The drawing under review shows one solid part. Ordinate dimensions are in mm from its lowest x, y, z. Round coordinates to 2 decimals unless told otherwise and drop trailing zeros. Write each loop counter-clockwise with the first axis right and the second up, starting at its lowest first coordinate (ties: lowest second). Pieces come first, ordered by that corner, then holes. Notation, with made-up numbers: (-32, -24.5) -> (19, -24.5) arc R29 ccw to (19, 9.5) -> close; hole circle Ø3 at (39.25, -19). An arc over 180 degrees is marked (long way). Answer in a Markdown table with one row per item.
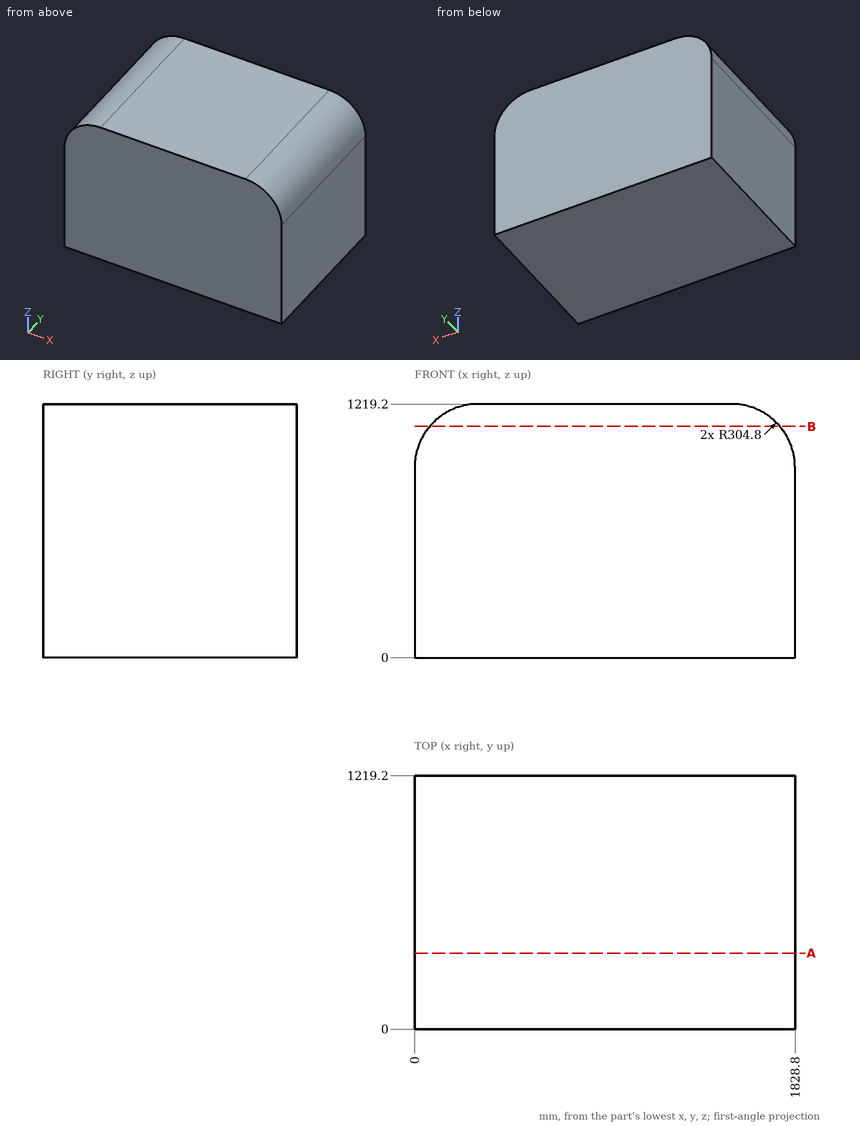
1) For line 1 (Z direction, x = 1564.5, y = 123); line 2 (X direction, y = 1023.5, z = 1138); line 3 (Z direction, x = 195.5, y = 501), list the stretches that pass through material, from the lowest coordinate up. Write a range as [from, to].
Solved:
| item | result |
|---|---|
| line 1 | [0, 1216.5] |
| line 2 | [97.66, 1731.14] |
| line 3 | [0, 1198.93] |
2) Consider section B-B on z = 1111.5. State the section outline as (x, y) points, then the cut area to 3 significant figures.
Solved:
| item | result |
|---|---|
| outline | (72.3, 0) -> (1756.5, 0) -> (1756.5, 1219.2) -> (72.3, 1219.2) -> close |
| area | 2,050,000 mm² |
3) Consider section A-A on y = 366. State the section outline as (x, z) points, then the cut area to 3 significant figures.
Solved:
| item | result |
|---|---|
| outline | (0, 0) -> (1828.8, 0) -> (1828.8, 914.4) arc R304.8 ccw to (1524, 1219.2) -> (304.8, 1219.2) arc R304.8 ccw to (0, 914.4) -> close |
| area | 2,190,000 mm² |
